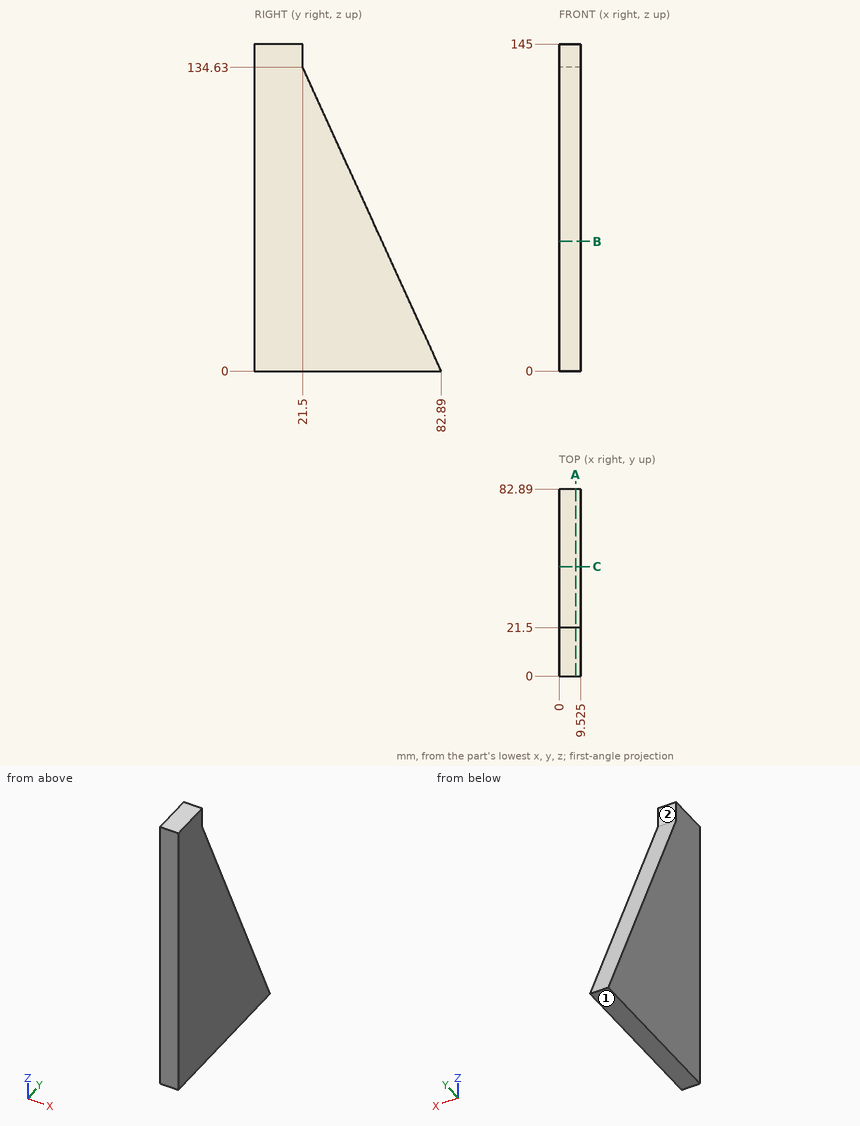
Geometry: see drawing. Coordinates: mm, zero at the bounding-box minimum. A direction names the side the tool comes from. Round coordinates to 2 decimals unless told otherwise and drop trailing zeros. Loops run counter-clockwise (first coordinate to the right, second up) from the corner with the lowest first, then second, coordinate; pieces in that order, holes last. Notation, with made-up numbers: M 23.25,14 L 58.25,14 A30 ccw 58.25,47 Z; hole C 57,11.25 d2. An arc over 180 degrees is marked long. Use a Markdown table: item, result. Add a question column.
1. Set-up query: the marked faces 1 and 2. Return all of +Z, -Z, +X, -X, +Y, -Y with unobstructed straight access to the full face (end or side cutting, diameter ignored); none if empty.
2. Cut plane B-B, the plane z = 57.5. Output: boundary loops of the cut face in (x, y) (3 decimals).
3. Cut plane A-A, the plane x = 7.25. Output: boundary loops of the cut face in (y, z).
4. Cut plane C-C, the plane y = 48.5. Output: boundary loops of the cut face in (x, z) (3 decimals).
5. Contact query for flat-ended pins moving along their axis: pin 1 (4 mm diameter, centred on x = 4.5, y = 52, fed in from +Z); pin 2 (2 mm diameter, centred on x = 3, y = 32.5, fed in from +Z). Output: stop coordinate, or through.
6. Ray query, line 1 along Y through (x, z) = (2, 137); line 2 along Z through (x, y) = (4, 27.5); line 3 along Y through (x, z) = (4, 10.5). Return the intervals inside material, ascending. Write a range as [from, to].
Solution:
| question | item | result |
|---|---|---|
| 1 | face 1 | -Z, +X, -X, +Y, -Y |
| 1 | face 2 | +Z, +X, -X, +Y |
| 2 | outline | M 0,0 L 9.525,0 L 9.525,56.671 L 0,56.671 Z |
| 3 | outline | M 0,0 L 82.89,0 L 21.5,134.63 L 21.5,145 L 0,145 Z |
| 4 | outline | M 0,0 L 9.525,0 L 9.525,75.418 L 0,75.418 Z |
| 5 | pin 1 | stops at z = 72.13 |
| 5 | pin 2 | stops at z = 112.7 |
| 6 | line 1 | y = [0, 21.5] |
| 6 | line 2 | z = [0, 121.47] |
| 6 | line 3 | y = [0, 78.1] |
